Verification items for this drawing (mm, ordinates from the low corner). A direction names the side the tool comes from. Give positions to 0.01 mm unless a question says otherwise; leave off trailing zeros. Loops run counter-clockwise (first coordinate to the right, second up) from the corner with the lowest first, then second, coordinate; pieces in that order, holes last. Notation, with made-up numbers: M -9.75,46 L 10.25,46 A24 ccw 10.25,78 Z; hole C -27,-32.75 d2. An arc over 180 degrees is marked long. Use one line per item in the form item = value.
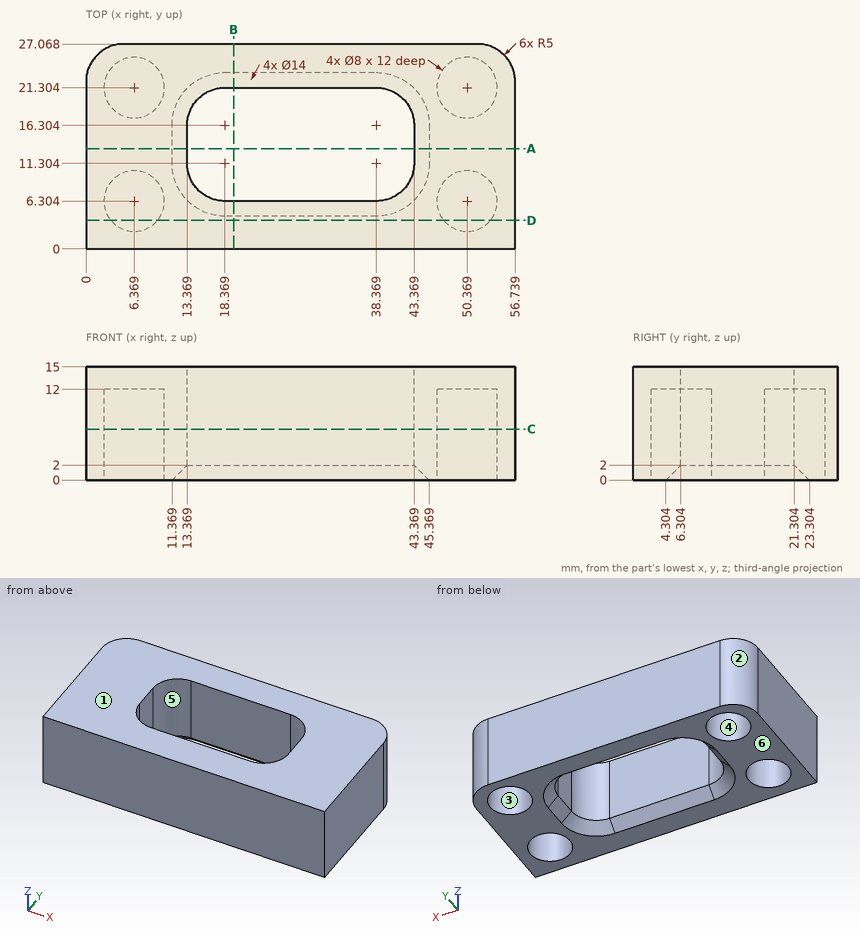
1) Scan lines: line 1 (Y direction, x = 48, z = 4); line 2 (Y direction, x = 52.5, z = 4); line 3 (Y direction, x = 19, z = 4). Record each from-to range of solid material in increasing order.
Evaluation:
line_1 = 0 to 3.08, 9.53 to 18.08, 24.53 to 27.07
line_2 = 0 to 2.92, 9.69 to 17.92, 24.69 to 27.01
line_3 = 0 to 6.3, 21.3 to 27.07
2) Depth check by flat-ended pin: pin 1 Ø1 at (x, y) = (31, 20) entering from -Z; pin 2 Ø2.5 at (x, y) = (49, 6) entering from -Z. Enter the tip coordinate at first touch or a pass-through.
Evaluation:
pin_1 = through
pin_2 = 12
3) Set-up check for the marked faces 4, 5 and 6: record each of +Z, -Z, +X, -X, +Y, -Y from which the full face is reachable in a straight line by a thin tool's end or side.
Evaluation:
face_4 = -Z
face_5 = +Z, -Z
face_6 = -Z, +X, -X, +Y, -Y
4) Section check C-C (z = 6.75). Record the cut outline in (x, y).
Evaluation:
outline = M 0,0 L 56.74,0 L 56.74,22.07 A5 ccw 51.74,27.07 L 5,27.07 A5 ccw 0,22.07 Z; hole C 6.37,6.3 d8; hole C 6.37,21.3 d8; hole M 13.37,11.3 A5 ccw 18.37,6.3 L 38.37,6.3 A5 ccw 43.37,11.3 L 43.37,16.3 A5 ccw 38.37,21.3 L 18.37,21.3 A5 ccw 13.37,16.3 Z; hole C 50.37,6.3 d8; hole C 50.37,21.3 d8
5) Section check A-A (y = 13.25). Record the cut outline in (x, z), then the cut area to 3 significant figures.
Evaluation:
outline = M 0,0 L 11.37,0 L 13.37,2 L 13.37,15 L 0,15 Z; M 43.37,2 L 45.37,0 L 56.74,0 L 56.74,15 L 43.37,15 Z
area = 397 mm^2
6) Section check B-B (x = 19.5). Record the cut outline in (y, z), then the cut area to 3 significant figures.
Evaluation:
outline = M 0,0 L 4.3,0 L 6.3,2 L 6.3,15 L 0,15 Z; M 21.3,2 L 23.3,0 L 27.07,0 L 27.07,15 L 21.3,15 Z
area = 177 mm^2
7) Section check D-D (y = 3.75). Record the cut outline in (x, z).
Evaluation:
outline = M 0,0 L 3.29,0 L 3.29,12 L 9.45,12 L 9.45,0 L 47.29,0 L 47.29,12 L 53.45,12 L 53.45,0 L 56.74,0 L 56.74,15 L 0,15 Z
8) Release check for a two-part mould opening along Y. For the marked faces 1, 2 and 3 record: pulls with the +Y half, pulls with the -Y half, needs draft (parallel to the pull), parting line crosses it, or undercut.
Evaluation:
face_1 = needs draft
face_2 = pulls with the +Y half
face_3 = undercut
